```python
from build123d import *

# Parameters (mm, degrees)
BOSS_EXTRUDE1_DEPTH = 5
SKETCH2_W           = 5
SKETCH2_H           = 14
SKETCH2_W_2         = 10
SKETCH2_H_2         = 5
SKETCH2_R           = 20
CUT_EXTRUDE1_DEPTH  = 210.418973113


with BuildPart() as part:
    # Sketch1 → Boss-Extrude1 (new body)
    with BuildSketch(Plane(origin=(0, 0, 0), x_dir=(1, 0, 0), z_dir=(0, 1, 0))):
        Polygon((-57.5, 167.947331922), (57.5, 167.947331922), (125, 37.947331922), (125, -0.052668078), (-125, -0.052668078), (-125, 37.947331922), align=None)
    extrude(amount=BOSS_EXTRUDE1_DEPTH)

    # Sketch2 → Cut-Extrude1 (cut, through all)
    with BuildSketch(Plane(origin=(0, 5, 0), x_dir=(1, 0, 0), z_dir=(0, 1, 0))):
        Polygon((-77.788864465, 128.872481842), (-103.476511391, 79.39997665), (-99.075067661, 77.027785029), (-73.843707474, 125.621215804), (-73.351788432, 126.56861544), align=None)
        Polygon((-125, 37.947331922), (-125, 23.947331922), (-120, 23.947331922), (-120, 36.728164098), (-103.683242772, 68.152835894), (-108.083917213, 70.526454327), align=None)
        with Locations((-122.5, 6.947331922)):
            Rectangle(SKETCH2_W, SKETCH2_H)
        with Locations((0, 45.447331922)):
            Rectangle(SKETCH2_W_2, SKETCH2_H_2)
        Polygon((-8.411070301, 132.656760174), (-13.226399097, 133.599762064), (-15.148227411, 123.786170675), (-10.332898614, 122.843168786), align=None)
        Polygon((10.332898614, 122.843168786), (15.148227411, 123.786170675), (13.226399097, 133.599762064), (8.411070301, 132.656760174), align=None)
        Polygon((-73.180711758, 137.74744261), (-68.74270223, 135.443091446), (-51.865499988, 167.947331922), (-57.5, 167.947331922), align=None)
        Polygon((73.351788432, 126.56861544), (73.843707474, 125.621215804), (99.075067661, 77.027785029), (103.476511391, 79.39997665), (77.788864465, 128.872481842), align=None)
        Polygon((68.74270223, 135.443091446), (73.180711758, 137.74744261), (57.5, 167.947331922), (51.865499988, 167.947331922), align=None)
        with Locations((122.5, 6.947331922)):
            Rectangle(SKETCH2_W, SKETCH2_H)
        Polygon((125, 23.947331922), (125, 37.947331922), (108.083917213, 70.526454327), (103.683242772, 68.152835894), (120, 36.728164098), (120, 23.947331922), align=None)
        with Locations(Location((0, 72.947331922, 0), (0, 0, 270))):
            Circle(SKETCH2_R)
    extrude(amount=-CUT_EXTRUDE1_DEPTH, mode=Mode.SUBTRACT)


solid = part.part
```
Input: part model. Units: mm. Frame: model coordinates. A direction names the side the tool comes from. Round coordinates to 2 decimals unless told otherwise and drop trailing zeros. Loops run counter-clockwise (first coordinate to the right, second up) from the corner with the lowest first, then second, coordinate; pieces in that order, holes last. Notation, with made-up numbers: (62.5, -38) -> (87.5, -38) arc R20 ccw to (87.5, 0) -> close; hole circle Ø11 at (-30.75, 63). An arc over 180 degrees is marked (long way). One line per item, written item: value.
(1) Pin query (flat end, axial travel): pin 1 (1.5 mm diameter, centred on y = 2, z = -46.5, fed in from +X); pin 2 (24 mm diameter, centred on x = 0, z = -72.95, fed in from +Y); pin 3 (2 mm diameter, centred on y = 2.5, z = -148.5, fed in from +X); pin 4 (1.5 mm diameter, centred on y = 3.5, z = -4, fed in from +X). Return the tip coordinate at first contact, or that it passes through.
Geometry check:
pin 1: x = 115.32
pin 2: through
pin 3: x = 62.48
pin 4: x = 120
(2) Mould query, pull axis Z, two halves, no side actions, for faces 1 (the face through (-9.385, 2.535, -127.681)), 2 (the face through (14.2, 2.54, -128.62)), 3 (the face through (75.453, 2.465, -133.372)), 4 (the face through (120, 3, -7)). Classes: pulls with the +Z half, pulls with the -Z half, needs draft (parallel to the pull), parting line crosses it, or undercut.
Geometry check:
face 1: undercut
face 2: undercut
face 3: pulls with the -Z half
face 4: needs draft
(3) Section B-B (z = -74.5). Return the cut outline in (x, y), plus the area to 3 significant figures.
Geometry check:
outline: (-106.02, 0) -> (-19.94, 0) -> (-19.94, 5) -> (-106.02, 5) -> close; (19.94, 0) -> (106.02, 0) -> (106.02, 5) -> (19.94, 5) -> close
area: 861 mm2
(4) Set-up query: faces 5 (the face through (5, 3, -45)), 6 (the face through (-111.956, 2.535, -52.221)), 7 (the face through (-120, 3, -7)), 8 (the face through (122, 3, -13.947)). Return all of +Z, -Z, +X, -X, +Y, -Y with unobstructed straight access to the full face (end or side cutting, diameter ignored); none if empty.
Geometry check:
face 5: +Y, -Y
face 6: -X, +Y, -Y
face 7: +Z, -X, +Y, -Y
face 8: +Z, +X, +Y, -Y
(5) Section D-D (z = -105). Return the cut outline in (x, y).
Geometry check:
outline: (-84.55, 0) -> (84.55, 0) -> (84.55, 5) -> (-84.55, 5) -> close
(6) Material intervals for line 1 (X direction, y = 3, z = -132.5); line 2 (X direction, y = 2.5, z = -13); line 3 (Z direction, x = 17, y = 4.3), sorted ascending. Write a range as [from, to].
Geometry check:
line 1: [-75.91, -13.44], [-8.44, 8.44], [13.44, 75.91]
line 2: [-120, 120]
line 3: [-167.95, -83.48], [-62.41, 0.05]
(7) Section C-C (y = 1.65). Give the number of separate pieces and of enclosed holes in the cut face, plus the area to 3 significant figures.
Geometry check:
separate pieces: 1
enclosed holes: 4
area: 30,300 mm2
(8) Section A-A (x = 0). Return the cut outline in (y, z).
Geometry check:
outline: (0, -167.95) -> (5, -167.95) -> (5, -92.95) -> (0, -92.95) -> close; (0, -52.95) -> (5, -52.95) -> (5, -47.95) -> (0, -47.95) -> close; (0, -42.95) -> (5, -42.95) -> (5, 0.05) -> (0, 0.05) -> close
